from build123d import *

# Parameters (mm, degrees)
SKETCH_6_W      = 1.8
SKETCH_6_H      = 0.3
EXTRUDE_2_DEPTH = 3.5
CHAMFER_2_SIZE  = 1
CHAMFER_3_SIZE  = 0.4


with BuildPart() as part:
    # 草图1 → 旋转2 (revolve)
    with BuildSketch(Plane(origin=(0, 0, 0), x_dir=(0, 0, -1), z_dir=(1, 0, 0))):
        Polygon((-18.4, 0), (-18.4, 3.5), (-17, 3.5), (-17, 5.25), (-15, 5.25), (-15, 4), (-6, 4), (-6, 3.5), (0, 3.5), (0, 0), align=None)
    revolve(axis=Axis((0, 0, 0), (0, 0, 1)))

    # 草图6 → 凸台-拉伸2 (add)
    with BuildSketch(Plane(origin=(0, 0, 0), x_dir=(-1, 0, 0), z_dir=(0, 0, -1))):
        with Locations((0, 2.25)):
            Rectangle(SKETCH_6_W, SKETCH_6_H)
        with Locations((0, -2.25)):
            Rectangle(SKETCH_6_W, SKETCH_6_H)
    extrude(amount=EXTRUDE_2_DEPTH)

    # 倒角2
    chamfer_2_edges = [part.edges().sort_by_distance(p)[0] for p in [
        (0, -5.25, 17),
    ]]
    chamfer(chamfer_2_edges, length=CHAMFER_2_SIZE)

    # 倒角3
    chamfer_3_edges = [part.edges().sort_by_distance(p)[0] for p in [
        (-0.9, 2.25, -3.5),
        (0.9, 2.25, -3.5),
        (-0.9, -2.25, -3.5),
        (0.9, -2.25, -3.5),
    ]]
    chamfer(chamfer_3_edges, length=CHAMFER_3_SIZE)


solid = part.part
Input: part model. Units: mm. Frame: model coordinates. A direction names the side the tool comes from. Give positions to 0.01 mm unless a question says otherwise; leave off trailing zeros. Loops run counter-clockwise (first coordinate to the right, second up) from the corner with the lowest first, then second, coordinate; pieces in that order, holes last. Notation, with made-up numbers: (-20.5, -20) -> (29.5, -20) arc R4 cw to (29.5, -14) -> close; hole circle Ø8 at (20, -2). An arc over 180 degrees is marked (long way). Answer as a JSON object with one key per item and string values. Group by question number.
Item 1: Pull-direction query (Y, two-part tool) for faces 6 (the flat face through (0, 2.4, -2)), 7 (the flat face through (0, 2.1, -2)), 8 (the cylindrical face through (1.341, 3.233, 17.69)); classes: released by +Y, released by -Y, zero draft, split by the parting line, or undercut.
Item 2: Line query: probe 1 along Z at (x, y) = (-3.75, 0.5); probe 2 along Z at (x, y) = (-1, 0.25); probe 3 along Y at (x, z) = (-1, 9). Output: solid intervals per line, ascending.
Item 3: Cut plane A-A, the plane z = -0.75. Return the cut outline in (x, y).
Item 4: Cut plane D-D, the plane z = 3. Return the cut outline in (x, y).
Item 5: Reachability of faces 1 (the cylindrical face through (3.905, -0.867, 10.437)), 2 (the flat face through (0, 0, 18.4)), 3 (the flat face through (0, -2.4, -2)), 4 (the flat face through (0, -2.1, -2)), 5 (the cylindrical face through (-1.6, 5, 15.5)) from +Z, -Z, +X, -X, +Y, -Y: full face, straight path, thin tool, end or side. Return the list, or none.
Item 6: Cut plane B-B, the plane x = 0. Return the cut outline in (y, z).
Item 7: Pin query (flat end, axial travel): P1, Ø3, axis at x = 1, z = 11, coming from the -Y side; P2, Ø6, axis at y = -1.5, z = 9.5, coming from the -X side; P3, Ø1.5, axis at x = -2.5, y = -1.5, coming from the -Z side; P4, Ø2.5, axis at x = -0.5, y = 1, coming from the -Z side. Return the tip coordinate at first contact, or that it passes through.
Item 8: Cut plane C-C, the plane y = 0. Return the cut outline in (x, z), and give its area (3 significant figures).
Checks:
{
 "1": {"face 6": "released by +Y", "face 7": "undercut", "face 8": "split by the parting line"},
 "2": {"probe 1": "z = 6 to 17", "probe 2": "z = 0 to 18.4", "probe 3": "y = -3.87 to 3.87"},
 "3": {"outline": "(-0.9, -2.4) -> (0.9, -2.4) -> (0.9, -2.1) -> (-0.9, -2.1) -> close; (-0.9, 2.1) -> (0.9, 2.1) -> (0.9, 2.4) -> (-0.9, 2.4) -> close"},
 "4": {"outline": "circle Ø7 at (0, 0)"},
 "5": {"face 1": "-Z", "face 2": "+Z, +X, -X, +Y, -Y", "face 3": "-Z, +X, -X, -Y", "face 4": "-Z, +X, -X", "face 5": "+Z, -Z"},
 "6": {"outline": "(-5.25, 15) -> (-4, 15) -> (-4, 6) -> (-3.5, 6) -> (-3.5, 0) -> (-2.4, 0) -> (-2.4, -3.5) -> (-2.1, -3.5) -> (-2.1, 0) -> (2.1, 0) -> (2.1, -3.5) -> (2.4, -3.5) -> (2.4, 0) -> (3.5, 0) -> (3.5, 6) -> (4, 6) -> (4, 15) -> (5.25, 15) -> (5.25, 16) -> (4.25, 17) -> (3.5, 17) -> (3.5, 18.4) -> (-3.5, 18.4) -> (-3.5, 17) -> (-4.25, 17) -> (-5.25, 16) -> close"},
 "7": {"P1": "stops at y = -4", "P2": "stops at x = -4", "P3": "stops at z = 0", "P4": "stops at z = -3.5"},
 "8": {"outline": "(-5.25, 15) -> (-4, 15) -> (-4, 6) -> (-3.5, 6) -> (-3.5, 0) -> (3.5, 0) -> (3.5, 6) -> (4, 6) -> (4, 15) -> (5.25, 15) -> (5.25, 16) -> (4.25, 17) -> (3.5, 17) -> (3.5, 18.4) -> (-3.5, 18.4) -> (-3.5, 17) -> (-4.25, 17) -> (-5.25, 16) -> close", "area": "144 mm²"}
}
